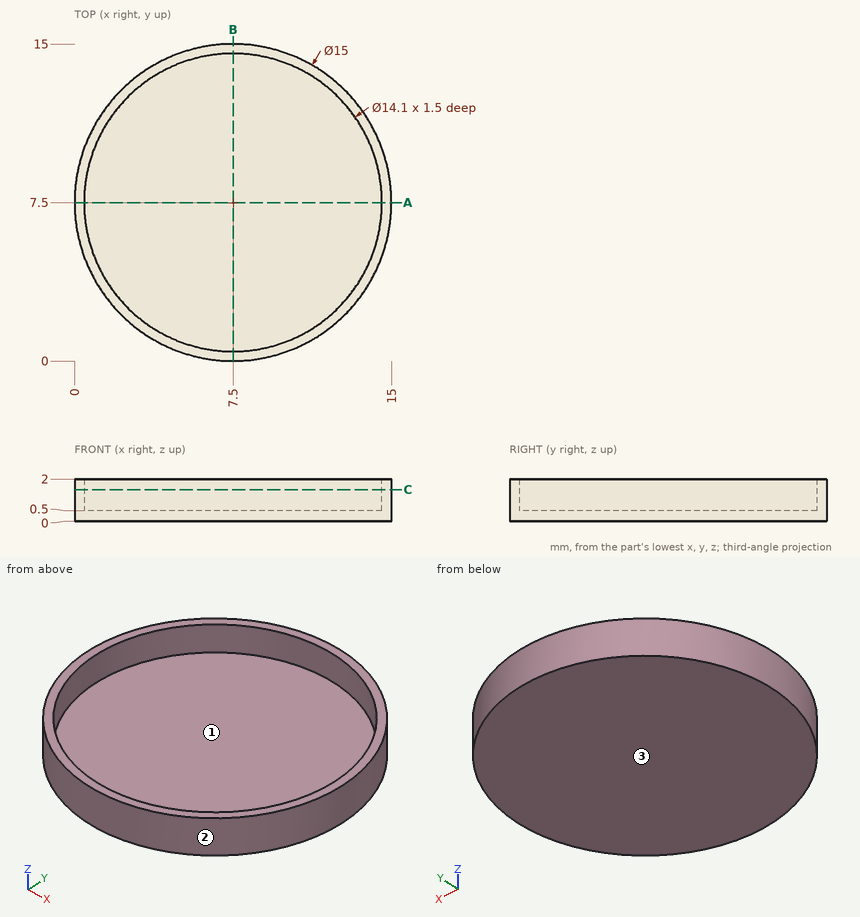
Geometry check sheet. Reference: drawing and pictorial views, mm from the part's lowest x, y, z. Round coordinates to 2 decimals unless told otherwise and drop trailing zeros. Order: outer loops, then holes, each group sorted by start corner. A loop starts at its lowest first (then second) coordinate and runs counter-clockwise, first axis right, second up. Notation, with made-up numbers: (76, 52) -> (129, 52) arc R12 ccw to (129, 63) -> close; hole circle Ø8 at (12, 17.5). An arc over 180 degrees is marked (long way). One line per item, written item: value. Start each with the question number.
Q1. Cross-section at A-A (y = 7.5). Record the boundary of the cut face in (x, z), and give its area (3 significant figures).
Q2. Cross-section at C-C (z = 1.5). Record the boundary of the cut face in (x, y).
Q3. Mould release check, pull along Y, two halves, no side actions. Record for the marked faces 1, 2 and 3: pulls with the +Y half, pulls with the -Y half, needs draft (parallel to the pull), parting line crosses it, or undercut.
Q4. Gauge pin test, flat ends, axial feed: pin 1 Ø1 at (y, z) = (11.5, 0.5) entering from +X; pin 2 Ø2 at (x, y) = (6, 9.5) entering from +Z; pin 3 Ø1 at (x, z) = (2.5, 0.5) entering from -Y. Record the tip position at first contact, or that the pin passes through.
Q5. Thickness scan on line 1 (Y direction, x = 7.5, z = 1.65); line 2 (Y direction, x = 4.75, z = 1.85). Record the ranges inside material, lowest first.
Completed:
1. outline: (0, 0) -> (15, 0) -> (15, 2) -> (14.55, 2) -> (14.55, 0.5) -> (0.45, 0.5) -> (0.45, 2) -> (0, 2) -> close
1. area: 8.85 mm²
2. outline: circle Ø15 at (7.5, 7.5); hole circle Ø14.1 at (7.5, 7.5)
3. face 1: undercut
3. face 2: parting line crosses it
3. face 3: needs draft
4. pin 1: stops at x = 14.13
4. pin 2: stops at z = 0.5
4. pin 3: stops at y = 1.5
5. line 1: y = 0 to 0.45, 14.55 to 15
5. line 2: y = 0.52 to 1.01, 13.99 to 14.48
